Autodesk Inventor part; units mm, degrees
ref_plane "YZ Plane" through (0, 0, 0) normal (1, 0, 0) x (0, 1, 0)
ref_plane "XZ Plane" through (0, 0, 0) normal (0, 1, 0) x (-1, 0, 0)
ref_plane "XY Plane" through (0, 0, 0) normal (0, 0, 1) x (1, 0, 0)
sketch "草圖1" plane through (0, 0, 0) normal (0, 1, 0) x (-1, 0, 0)
  circle A0 centre (0, 0) radius 70
  circle A1 centre (0, 0) radius 25
  line L0 (-70, 10) -> (-10, 10)
  line L1 (-10, 10) -> (-10, -10)
  line L2 (-10, -10) -> (-70, -10)
  line L3 (-70, -10) -> (-70, 10)
  line L4 (0, 0) -> (0, -55)
  line L5 (0, 0) -> (35.3533, -42.1324)
  arc A2 (0, -55) -> (35.3533, -42.1324) centre (0, 0) ccw
  line L6 (0, 0) -> (51.6831, -18.8111)
  line L7 (0, 0) -> (51.6831, 18.8111)
  arc A3 (51.6831, -18.8111) -> (51.6831, 18.8111) centre (0, 0) ccw
  line L8 (0, 0) -> (35.3533, 42.1324)
  line L9 (0, 0) -> (0, 55)
  arc A4 (35.3533, 42.1324) -> (0, 55) centre (0, 0) ccw
  circle A5 centre (0, 0) radius 2
  line L10 (-1.5, 1.3229) -> (-1.5, -1.3229)
  line L11 (-53.6, -11.7755) -> (-50.6, -11.7755)
  line L12 (-10, -11.7968) -> (-7, -11.7968)
  line L13 (-50.6, -11.8181) -> (-50.6, -15.8181)
  line L14 (-50.6, -15.8181) -> (-53.6, -15.8181)
  line L15 (-53.6, -15.8181) -> (-53.6, -11.8181)
  line L16 (-7, -11.7968) -> (-7, -15.7968)
  line L17 (-7, -15.7968) -> (-10, -15.7968)
  line L18 (-10, -15.7968) -> (-10, -11.7968)
  line L19 (-42.3, -47.9058) -> (-38.3, -47.9058)
  line L20 (-38.3, -47.9058) -> (-38.3, -50.9058)
  line L21 (-38.3, -50.9058) -> (-42.3, -50.9058)
  line L22 (-42.3, -50.9058) -> (-42.3, -47.9058)
  line L23 (-22.3, -47.9058) -> (-18.3, -47.9058)
  line L24 (-18.3, -47.9058) -> (-18.3, -50.9058)
  line L25 (-18.3, -50.9058) -> (-22.3, -50.9058)
  line L26 (-22.3, -50.9058) -> (-22.3, -47.9058)
  line L27 (-10, -10) -> (-10, -11.349)
  line L28 (-50.6, -11.8181) -> (-53.6, -11.8181)
  line L29 (-53.6, -11.8181) -> (-53.6, -15.8181)
  line L30 (-50.6, -15.8181) -> (-50.6, -11.8181)
  line L31 (-4, -24) -> (-4, -21) construction
  line L32 (-10, -21) -> (-6, -21) construction
  line L33 (-6, -21) -> (-4, -21) construction
  line L34 (-6, -24) -> (-4, -24) construction
  line L35 (-10, -24) -> (-6, -24) construction
  line L36 (-12, -24) -> (-12, -21) construction
  line L37 (-6, -21) -> (-10, -21)
  line L38 (-10, -21) -> (-10, -24)
  line L39 (-10, -24) -> (-6, -24)
  line L40 (-6, -24) -> (-6, -21)
  line L41 (-50.6, -24) -> (-54.6, -24)
  line L42 (-54.6, -24) -> (-54.6, -21)
  line L43 (-54.6, -21) -> (-50.6, -21)
  line L44 (-50.6, -21) -> (-50.6, -24)
  line L45 (-10, -16.4) -> (-10, -21)
  point P0 (-23, -10)
  point P1 (16.0697, -19.1511)
  point P2 (0, -25)
  point P3 (-69.282, 10)
  point P4 (-69.282, -10)
  point P5 (16.0697, 19.1511)
  point P6 (0, 25)
  point P7 (23.4923, -8.5505)
  point P8 (23.4923, 8.5505)
  point P9 (-70, 0)
  point P10 (-10, 0)
  point P11 (-23, -7)
  point P12 (-52.6, -24)
  point P13 (-8, -24)
  point P14 (-22.9129, 10)
  point P15 (-22.9129, -10)
  dimension "d0" = 140
  dimension "d1" = 50
  dimension "d2" = 20
  dimension "d3" = 60
  dimension "d5" = 40
  dimension "d6" = 55
  dimension "d9" = 140
  dimension "d28" = 4
  dimension "d29" = 1.5
  dimension "d32" = 13
  dimension "d57" = 1.349
  dimension "d58" = 40.6
  dimension "d59" = 4.6
extrude "擠出1" add sketch "草圖1" along normal blind 3 contours A0 L2 A1 L38 L39 L4 A2 L5 L6 A3 L7 L8 A4 L9 L0 | L0 L1 L2 A1 | A1 L9 A5 L4 L39 L40 L37 L38 L2 L1 L0 | A1 L8 A5 L9 | A1 L7 A5 L8 | A1 L6 A5 L7 | L4 A5 L5 A1 | A5 L6 A1 L5
sketch "草圖2" plane through (0, 3, 0) normal (0, 1, 0) x (1, 0, 0)
  line L0 (-3, 13) -> (3, 13)
  line L1 (3, 13) -> (3, 10)
  line L2 (3, 10) -> (-3, 10)
  line L3 (-3, 10) -> (-3, 13)
  line L4 (-12.7583, 3.9019) -> (-9.7583, 9.0981)
  line L5 (-9.7583, 9.0981) -> (-7.1603, 7.5981)
  line L6 (-7.1603, 7.5981) -> (-10.1603, 2.4019)
  line L7 (-10.1603, 2.4019) -> (-12.7583, 3.9019)
  line L8 (-9.7583, -9.0981) -> (-12.7583, -3.9019)
  line L9 (-12.7583, -3.9019) -> (-10.1603, -2.4019)
  line L10 (-10.1603, -2.4019) -> (-7.1603, -7.5981)
  line L11 (-7.1603, -7.5981) -> (-9.7583, -9.0981)
  line L12 (3, -13) -> (-3, -13)
  line L13 (-3, -13) -> (-3, -10)
  line L14 (-3, -10) -> (3, -10)
  line L15 (3, -10) -> (3, -13)
  line L16 (-66, 3) -> (-63, 3)
  line L17 (-63, 3) -> (-63, -3)
  line L18 (-63, -3) -> (-66, -3)
  line L19 (-66, -3) -> (-66, 3)
  line L20 (-34.0981, -53.0596) -> (-28.9019, -56.0596)
  line L21 (-28.9019, -56.0596) -> (-30.4019, -58.6577)
  line L22 (-30.4019, -58.6577) -> (-35.5981, -55.6577)
  line L23 (-35.5981, -55.6577) -> (-34.0981, -53.0596)
  line L24 (28.9019, -56.0596) -> (34.0981, -53.0596)
  line L25 (34.0981, -53.0596) -> (35.5981, -55.6577)
  line L26 (35.5981, -55.6577) -> (30.4019, -58.6577)
  line L27 (30.4019, -58.6577) -> (28.9019, -56.0596)
  line L28 (63, -3) -> (63, 3)
  line L29 (63, 3) -> (66, 3)
  line L30 (66, 3) -> (66, -3)
  line L31 (66, -3) -> (63, -3)
  line L32 (34.0981, 53.0596) -> (28.9019, 56.0596)
  line L33 (28.9019, 56.0596) -> (30.4019, 58.6577)
  line L34 (30.4019, 58.6577) -> (35.5981, 55.6577)
  line L35 (35.5981, 55.6577) -> (34.0981, 53.0596)
  line L36 (-28.9019, 56.0596) -> (-34.0981, 53.0596)
  line L37 (-34.0981, 53.0596) -> (-35.5981, 55.6577)
  line L38 (-35.5981, 55.6577) -> (-30.4019, 58.6577)
  line L39 (-30.4019, 58.6577) -> (-28.9019, 56.0596)
  point P0 (0, 0)
  point P1 (0, 10)
  point P2 (-8.6603, 5)
  point P3 (-8.6603, -5)
  point P4 (0, -10)
  point P5 (-63, 0)
  point P6 (-31.5, -54.5596)
  point P7 (31.5, -54.5596)
  point P8 (63, 0)
  point P9 (31.5, 54.5596)
  point P10 (-31.5, 54.5596)
  dimension "d33" = 3
  dimension "d34" = 6
  dimension "d35" = 10
  dimension "d38" = 180
  dimension "d49" = 3
  dimension "d50" = 6
  dimension "d51" = 63
  dimension "d54" = 360
extrude "擠出2" cut sketch "草圖2" against normal through all contours L0 L1 L2 L3 | L4 L5 L6 L7 | L8 L9 L10 L11 | L12 L13 L14 L15 | L16 L17 L18 L19 | L20 L21 L22 L23 | L24 L25 L26 L27 | L32 L33 L34 L35 | L36 L37 L38 L39
Here's how the part is built. I have some questions about the finished solid (model axes, mm). Coordinates: 2 decimals unless noted, no trailing zeros. Write each loop counter-clockwise with the first axis right and the second up, starting at its lowest first coordinate (ties: lowest second). Pieces come first, ordered by that corner, then holes. Notation, with made-up numbers: (72, -12.75) - (83, -12.75) arc R24 ccw to (83, 12.25) - close; hole circle Ø1 at (-5.75, -11.5). An arc over 180 degrees is marked (long way). Use one line per item in the form item = value.
1) I'm going to push flat-ended pins straight in: P1, Ø1.5, axis at y = 1.5, z = 11.5, coming from the -X side; P2, Ø1.5, axis at x = 51.5, y = 1.5, coming from the -Z side; P3, Ø0.9, axis at x = -65, y = 2, coming from the +Z side; P4, Ø8, axis at x = -5.5, z = -30, coming from the +Y side. Where does each tip first touch, or does it pass through?
Solved:
P1 = -69.17
P2 = -48.21
P3 = 27.08
P4 = through
2) Suppose I cut it at A-A, the plane z = -28. Write out the boundary of the cut face in (x, y).
Solved:
outline = (-64.16, 0) - (-23.49, 0) - (-23.49, 3) - (-64.16, 3) - close; (0, 0) - (64.16, 0) - (64.16, 3) - (0, 3) - close
3) I need wall thicknesses on line 1 (Z direction, x = -11, y = 1.95); line 2 (Z direction, x = 32, y = 0.3); line 3 (Z direction, x = -20, y = 0.6). Which ranges of each line are inside material? Lowest first, please.
Solved:
line_1 = -69.13 to -53.89, -22.45 to -6.95, -2.89 to 2.89, 6.95 to 22.45, 53.89 to 69.13
line_2 = -62.26 to -57.74, -54.27 to -10, 10 to 54.27, 57.74 to 62.26
line_3 = -67.08 to -51.23, -23.84 to 23.84, 51.23 to 67.08
4) Suppose I cut it at B-B, the plane x = -42.5. Write out the boundary of the cut face in (y, z).
Solved:
outline = (0, -55.62) - (3, -55.62) - (3, -15.47) - (0, -15.47) - close; (0, 15.47) - (3, 15.47) - (3, 55.62) - (0, 55.62) - close
5) Suppose I cut it at C-C, the plane y = 2.35. Give the number of separate pieces and of enclosed holes in the cut face, plus the area to 3 significant figures.
Solved:
separate_pieces = 1
enclosed_holes = 19
area = 11,700 mm2
